Input: part model. Units: mm. Frame: model coordinates. Face numbers are marked on the shaded views. A direction names the side the tool comes from. Round coordinates to 2 decimals unless told otherwise and drop trailing zeros. Loops run counter-clockwise (first coordinate to the right, second up) from the corner with the lowest first, then second, coordinate; pieces in that order, holes last. Notation, with made-up numbers: M 32,59 L 66,59 A11 ccw 66,79 Z; hole C 23.5,-18.5 d1. An arc over 180 degrees is marked long. Put each result on its own line as item: value. Start each with the question number.
1) Section C-C on z = 2.25. Output: boundary loops of the cut face in (x, y).
2) Draft query along X for the marked faces 1, 2 and 3. Return one class per face: +X half, -X half, draft (parallel to the pull), parting line (faces both ways), or undercut.
3) Line query: probe 1 along Y at (x, z) = (-17, 8.5); probe 2 along Z at (x, y) = (-1.5, 22.5); probe 3 along X at (y, z) = (28, 9). Output: solid intervals per line, ascending.
4) Reachability of the marked faces 4 and 5 from +Z, -Z, +X, -X, +Y, -Y: full face, straight path, thin tool, end or side. Return the list, or none.
5) Section A-A on z = 10. Output: boundary loops of the cut face in (x, y).
6) Pin query (flat end, axial travel): pin 1 (3 mm diameter, centred on x = 5, z = 4.5, fed in from +Y); pin 2 (2.5 mm diameter, centred on x = -19, y = -25.5, fed in from +Z); pin 3 (4 mm diameter, centred on x = 20, z = 11.5, fed in from -Y). Return the tip coordinate at first contact, or that it passes through.
7) Section D-D on y = -3. Output: boundary loops of the cut face in (x, z), plus the area to 3 significant figures.
8) Section B-B on z = 6.25. Output: boundary loops of the cut face in (x, y).
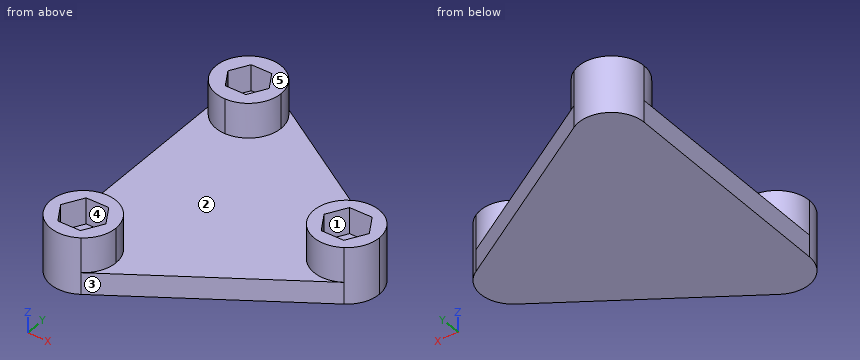
from build123d import *

# Parameters (mm, degrees)
F1_DEPTH = 5
F2_DEPTH = 13
F3_DEPTH = 7


with BuildPart() as f1:
    # F0 (on Top) → F1 (new body)
    with BuildSketch(Plane.XY):
        with BuildLine():
            ThreePointArc((-21.353622, 18.730685), (-26.656923, 20.927384), (-28.853622, 26.230685))
            Line((-28.853622, 26.230685), (-28.853622, -26.230685))
            ThreePointArc((-28.853622, -26.230685), (-26.656923, -20.927384), (-21.353622, -18.730685))
            Line((-21.353622, -18.730685), (-21.353622, 18.730685))
        make_face()
        with BuildLine():
            ThreePointArc((24.153526, -6.339776), (12.646378, 0), (24.153527, 6.339776))
            Line((24.153527, 6.339776), (-17.346473, 32.570461))
            ThreePointArc((-17.346473, 32.570461), (-14.784619, 29.849828), (-13.853622, 26.230685))
            ThreePointArc((-13.853622, 26.230685), (-16.050321, 20.927384), (-21.353622, 18.730685))
            Line((-21.353622, 18.730685), (-21.353622, -18.730685))
            ThreePointArc((-21.353622, -18.730685), (-16.050321, -20.927384), (-13.853622, -26.230685))
            ThreePointArc((-13.853622, -26.230685), (-14.784619, -29.849828), (-17.346473, -32.570461))
            Line((-17.346473, -32.570461), (24.153526, -6.339776))
        make_face()
    extrude(amount=F1_DEPTH)

    # F0 (on Top) → F2 (join)
    with BuildSketch(Plane.XY):
        with BuildLine():
            ThreePointArc((-28.853622, -26.230685), (-24.972765, -32.799689), (-17.346473, -32.570461))
            ThreePointArc((-17.346473, -32.570461), (-14.784619, -29.849828), (-13.853622, -26.230685))
            ThreePointArc((-13.853622, -26.230685), (-16.050321, -20.927384), (-21.353622, -18.730685))
            ThreePointArc((-21.353622, -18.730685), (-26.656923, -20.927384), (-28.853622, -26.230685))
        make_face()
        Polygon((-23.951698, -21.730685), (-21.353622, -21.730685), (-18.755546, -21.730685), (-16.15747, -26.230685), (-18.755546, -30.730685), (-23.951698, -30.730685), (-26.549775, -26.230685), align=None, mode=Mode.SUBTRACT)
        with BuildLine():
            ThreePointArc((24.153526, -6.339776), (26.715381, -3.619143), (27.646378, 0))
            ThreePointArc((27.646378, 0), (26.715381, 3.619143), (24.153527, 6.339776))
            ThreePointArc((24.153527, 6.339776), (12.646378, 0), (24.153526, -6.339776))
        make_face()
        Polygon((25.34253, 0), (22.744454, -4.5), (17.548302, -4.5), (14.950225, 0), (17.548302, 4.5), (22.744454, 4.5), align=None, mode=Mode.SUBTRACT)
        with BuildLine():
            ThreePointArc((-13.853622, 26.230685), (-14.784619, 29.849828), (-17.346473, 32.570461))
            ThreePointArc((-17.346473, 32.570461), (-24.972765, 32.799689), (-28.853622, 26.230685))
            ThreePointArc((-28.853622, 26.230685), (-26.656923, 20.927384), (-21.353622, 18.730685))
            ThreePointArc((-21.353622, 18.730685), (-16.050321, 20.927384), (-13.853622, 26.230685))
        make_face()
        Polygon((-18.983858, 22.126133), (-21.353622, 22.126133), (-23.723387, 22.126133), (-26.093151, 26.230685), (-23.723387, 30.335237), (-18.983858, 30.335237), (-16.614093, 26.230685), align=None, mode=Mode.SUBTRACT)
    extrude(amount=F2_DEPTH)

    # F0 (on Top) → F3 (join)
    with BuildSketch(Plane.XY):
        Polygon((-23.723387, 22.126133), (-21.353622, 22.126133), (-18.983858, 22.126133), (-16.614093, 26.230685), (-18.983858, 30.335237), (-23.723387, 30.335237), (-26.093151, 26.230685), align=None)
        Polygon((-18.755546, -21.730685), (-21.353622, -21.730685), (-23.951698, -21.730685), (-26.549775, -26.230685), (-23.951698, -30.730685), (-18.755546, -30.730685), (-16.15747, -26.230685), align=None)
        Polygon((17.548302, -4.5), (22.744454, -4.5), (25.34253, 0), (22.744454, 4.5), (17.548302, 4.5), (14.950225, 0), align=None)
    extrude(amount=F3_DEPTH)


solid = f1.part
Geometry results:
1. outline: M -28.85,-26.23 A7.5 ccw -17.35,-32.57 L 24.15,-6.34 A7.5 ccw 27.65,0 A7.5 ccw 24.15,6.34 L -17.35,32.57 A7.5 ccw -28.85,26.23 Z
2. face 1: undercut
2. face 2: draft
2. face 3: +X half
3. probe 1: y = -32.34 to -27.69, -24.77 to -20.12, 20.12 to 25.56, 26.9 to 32.34
3. probe 2: z = 0 to 5
3. probe 3: x = -28.64 to -25.07, -17.64 to -14.07
4. face 4: +Z
4. face 5: +Z, +X, -X, +Y, -Y
5. outline: M -28.85,-26.23 A7.5 ccw -17.35,-32.57 A7.5 ccw -13.85,-26.23 A7.5 ccw Z; M -28.85,26.23 A7.5 ccw -13.85,26.23 A7.5 ccw -17.35,32.57 A7.5 ccw Z; M 24.15,6.34 A7.5 ccw long 27.65,0 A7.5 ccw Z; hole M -26.55,-26.23 L -23.95,-30.73 L -18.76,-30.73 L -16.16,-26.23 L -18.76,-21.73 L -23.95,-21.73 Z; hole M -26.09,26.23 L -23.72,22.13 L -18.98,22.13 L -16.61,26.23 L -18.98,30.34 L -23.72,30.34 Z; hole M 14.95,0 L 17.55,-4.5 L 22.74,-4.5 L 25.34,0 L 22.74,4.5 L 17.55,4.5 Z
6. pin 1: stops at y = 19.39
6. pin 2: stops at z = 7
6. pin 3: stops at y = -7.5
7. outline: M -28.85,0 L 27.02,0 L 27.02,13 L 23.61,13 L 23.61,7 L 16.68,7 L 16.68,13 L 13.27,13 L 13.27,5 L -28.85,5 Z
7. area: 348 mm²
8. outline: M -28.85,-26.23 A7.5 ccw -17.35,-32.57 A7.5 ccw -13.85,-26.23 A7.5 ccw Z; M -28.85,26.23 A7.5 ccw -13.85,26.23 A7.5 ccw -17.35,32.57 A7.5 ccw Z; M 24.15,6.34 A7.5 ccw long 27.65,0 A7.5 ccw Z
